from build123d import *

# Parameters (mm, degrees)
F0_R     = 2.4
F1_DEPTH = 15
F2_W     = 2.267002
F2_H     = 3.049704
F3_DEPTH = 5


with BuildPart() as f1:
    # F0 (on Front) → F1 (new body)
    with BuildSketch(Plane.XZ):
        Circle(F0_R)
    extrude(amount=F1_DEPTH)

    # F2 (on face) → F3 (cut)
    with BuildSketch(Plane.XZ.offset(15)):
        Rectangle(F2_W, F2_H)
    extrude(amount=-F3_DEPTH, mode=Mode.SUBTRACT)


solid = f1.part
The model under review builds one solid part; all positions refer to its coordinate system, in mm. A direction names the side the tool comes from. Give positions to 0.01 mm unless a question says otherwise; leave off trailing zeros. Loops run counter-clockwise (first coordinate to the right, second up) from the corner with the lowest first, then second, coordinate; pieces in that order, holes last. Notation, with made-up numbers: (65.25, 84.25) -> (107.25, 84.25) arc R22 ccw to (107.25, 122.25) -> close; hole circle Ø9 at (21, 7). An arc over 180 degrees is marked (long way). Answer as a JSON object with one key per item and string values. Group by question number.
Q1. Draft analysis for pull direction Z (two halves, no side actions). For faces 3 (the flat face through (0, -10, 0)), 4 (the flat face through (0, 0, 0)), 5 (the cylindrical face through (1.29, -7.395, 2.024)), state which applies: pulls with the +Z half, pulls with the -Z half, needs draft (parallel to the pull), parting line crosses it, or undercut.
Q2. Wall thickness on line 1 along Y through (x, z) = (0.9, 0.65); line 2 along X through (y, z) = (-10.25, 0.85); line 3 along Z through (x, y) = (1.45, -9.25): over which ranges is each line inside the solid? List them lowest first.
Q3. Take a section at C-C (z = 0). Write out the cut boundary in (x, y).
Q4. Take a section at B-B (x = 0). Write out the cut boundary in (y, z).
Q5. Take a section at D-D (y = -4.25). Write out the cut boundary in (x, z).
Q6. Tool access review of faces 1 (the flat face through (0, -15, -2)), 2 (the flat face through (0, -13, -1.525)): name each direction out of +Z, -Z, +X, -X, +Y, -Y from which nothing blocks a thin tool from reaching the whole face with its end or side.
Q7. Take a section at A-A (y = -10.25). Write out the cut boundary in (x, z).
Q8. Insertion check: pin 1 (1.8 mm diameter, centred on x = 0.5, y = -13, fed in from -Z); pin 2 (0.7 mm diameter, centred on x = -0.5, y = -11.5, fed in from +Z). Each pin has a flat end and moves straight along its axis. Give the tip position at first contact, or say it passes through.
Answer below:
{
 "1": {"face 3": "undercut", "face 4": "needs draft", "face 5": "parting line crosses it"},
 "2": {"line 1": "y = -10 to 0", "line 2": "x = -2.24 to -1.13, 1.13 to 2.24", "line 3": "z = -1.91 to 1.91"},
 "3": {"outline": "(-2.4, -15) -> (-1.13, -15) -> (-1.13, -10) -> (1.13, -10) -> (1.13, -15) -> (2.4, -15) -> (2.4, 0) -> (-2.4, 0) -> close"},
 "4": {"outline": "(-15, -2.4) -> (0, -2.4) -> (0, 2.4) -> (-15, 2.4) -> (-15, 1.52) -> (-10, 1.52) -> (-10, -1.52) -> (-15, -1.52) -> close"},
 "5": {"outline": "circle Ø4.8 at (0, 0)"},
 "6": {"face 1": "+Z, -Z, +X, -X, -Y", "face 2": "-Y"},
 "7": {"outline": "circle Ø4.8 at (0, 0); hole (-1.13, -1.52) -> (1.13, -1.52) -> (1.13, 1.52) -> (-1.13, 1.52) -> close"},
 "8": {"pin 1": "stops at z = -2.4", "pin 2": "stops at z = 2.4"}
}
